from build123d import *

# Parameters (mm, degrees)
F0_W      = 117.348
F0_H      = 50.8
F1_DEPTH  = 25.4
F3_DEPTH  = 9.652
F2_R      = 9.525
F4_DEPTH  = 35.053
F5_W      = 60.452
F5_H      = 35.052
F6_DEPTH  = 12.7
F7_W      = 76.2
F7_H      = 17.526
F8_DEPTH  = 12.7
F9_W      = 41.148
F9_H      = 35.052
F10_DEPTH = 19.304


with BuildPart() as f1:
    # F0 (on Front) → F1 (new body)
    with BuildSketch(Plane.XZ):
        with Locations((19.444794, -1.353553)):
            Rectangle(F0_W, F0_H)
    extrude(amount=F1_DEPTH)

    # F0 (on Front) → F3 (join)
    with BuildSketch(Plane.XZ):
        with Locations((19.444794, -1.353553)):
            Rectangle(F0_W, F0_H)
    extrude(amount=-F3_DEPTH)

    # F2 (on face) → F4 (cut, through all)
    with BuildSketch(Plane.XZ.offset(25.4)):
        with Locations((-7.913983, -7.957553)):
            Circle(F2_R)
    extrude(amount=-F4_DEPTH, mode=Mode.SUBTRACT)

    # F5 (on face) → F6 (join)
    with BuildSketch(Plane(origin=(0, 0, -26.753553), x_dir=(1, 0, 0), z_dir=(0, 0, -1))):
        with Locations((47.892794, 25.4)):
            Rectangle(F5_W, F5_H)
    extrude(amount=F6_DEPTH)

    # F7 (on face) → F8 (cut)
    with BuildSketch(Plane.XY.offset(24.046447)):
        with Locations((-1.129206, -16.637)):
            Rectangle(F7_W, F7_H)
    extrude(amount=-F8_DEPTH, mode=Mode.SUBTRACT)

    # F9 (on face) → F10 (cut)
    with BuildSketch(Plane.XY.offset(24.046447)):
        with Locations((57.544794, -7.874)):
            Rectangle(F9_W, F9_H)
    extrude(amount=-F10_DEPTH, mode=Mode.SUBTRACT)


solid = f1.part
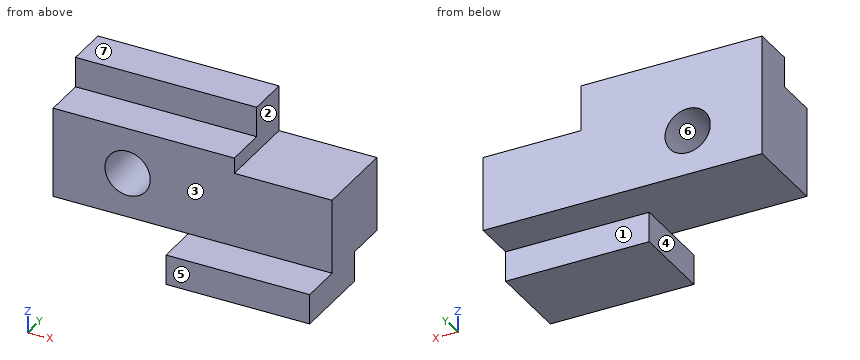
The listing builds one solid part. Answer for the finished solid, in the listing's coordinates (mm). Face numbers are marked on the shaded views. A direction names the side the tool comes from. Give positions to 0.01 mm unless a question says otherwise; leave off trailing zeros. Loops run counter-clockwise (first coordinate to the right, second up) from the corner with the lowest first, then second, coordinate; pieces in that order, holes last. Notation, with made-up numbers: (25, 40.5) - (35, 40.5) arc R18 cw to (35, 46.5) - close; hole circle Ø1 at (3.25, 69.25). An arc over 180 degrees is marked (long way). Use one line per item in the form item = value.
1. Given pin 1 Ø1.5 at (x, z) = (-23, -22) entering from -Y; pin 2 Ø15.5 at (y, z) = (-16.5, 14.5) entering from +X; pin 3 Ø14 at (y, z) = (-28.5, -30.5) entering from -X; pin 4 Ø5 at (x, y) = (-14.5, -14.5) entering from +Z, each flat-ended and moving along its own axis, determine where each tip first touches the part or whether it passes through.
Calculated:
pin_1 = -25.4
pin_2 = 36.97
pin_3 = -39.23
pin_4 = 11.35
2. Section D-D on z = -28 is taken. Give the vertices of the cut face in (x, y), then the cut area to 3 significant figures.
Calculated:
outline = (17.67, -42.93) - (78.12, -42.93) - (78.12, -7.87) - (17.67, -7.87) - close
area = 2,120 mm^2
3. The mould has two halves that part along Z. Classify the marked faces 5, 6 and 7: pulls with the +Z half, pulls with the -Z half, needs draft (parallel to the pull), parting line crosses it, or undercut.
Calculated:
face_5 = needs draft
face_6 = undercut
face_7 = pulls with the +Z half
4. Which of the six approach directions +Z, -Z, +X, -X, +Y, -Y give full straight-line access (tool end or side, diameter ignored) to the marked faces 1, 2, 3 and 4?
Calculated:
face_1 = -Z, +X, -X, +Y
face_2 = +Z, +X, +Y, -Y
face_3 = +Z, +X, -X, -Y
face_4 = -Z, -X, +Y, -Y
5. Section A-A on x = 27 is taken. Give the vertices of the cut face in (y, z).
Calculated:
outline = (-42.93, -39.45) - (-7.87, -39.45) - (-7.87, -26.75) - (9.65, -26.75) - (9.65, 24.05) - (-7.87, 24.05) - (-7.87, 11.35) - (-25.4, 11.35) - (-25.4, -26.75) - (-42.93, -26.75) - close
6. Section C-C on y = -13 is taken. Give the vertices of the cut face in (x, z) (3 decimals).
Calculated:
outline = (-39.229, -26.754) - (17.667, -26.754) - (17.667, -39.454) - (78.119, -39.454) - (78.119, 4.742) - (36.971, 4.742) - (36.971, 11.346) - (-39.229, 11.346) - close; hole circle Ø19.05 at (-7.914, -7.958)
7. Section B-B on z = -12 is taken. Give the vertices of the cut face in (x, y).
Calculated:
outline = (-39.23, -25.4) - (-16.54, -25.4) - (-16.54, 9.65) - (-39.23, 9.65) - close; (0.71, -25.4) - (78.12, -25.4) - (78.12, 9.65) - (0.71, 9.65) - close
8. Find the intervals of material crossed by line 1 along Y through (x, z) = (73.5, -16); line 2 along X through (y, z) = (-11, 11); line 3 along Z through (x, y) = (46, -33), in increasing order. Write a range as [from, to].
Calculated:
line_1 = [-25.4, 9.65]
line_2 = [-39.23, 36.97]
line_3 = [-39.45, -26.75]
